from build123d import *

# Parameters (mm, degrees)
SKETCH1_W           = 40
SKETCH1_H           = 40
BOSS_EXTRUDE1_DEPTH = 3.18
SKETCH2_W           = 3.18
SKETCH2_H           = 10
BOSS_EXTRUDE2_DEPTH = 60
SKETCH3_W           = 3.18
SKETCH3_H           = 16
BOSS_EXTRUDE3_DEPTH = 36
FILLET1_R           = 10
FILLET2_R           = 8
FILLET3_R           = 5
FILLET4_R           = 4
SKETCH7_R           = 1
CUT_EXTRUDE2_DEPTH  = 3.18
SKETCH8_R           = 1
CUT_EXTRUDE3_DEPTH  = 3.18


with BuildPart() as part:
    # Sketch1 → Boss-Extrude1 (new body)
    with BuildSketch(Plane.XY):
        with Locations((50, 0)):
            Rectangle(SKETCH1_W, SKETCH1_H)
    extrude(amount=BOSS_EXTRUDE1_DEPTH)

    # Sketch2 → Boss-Extrude2 (add)
    with BuildSketch(Plane.ZY.offset(-30)):
        with Locations((1.59, 0)):
            Rectangle(SKETCH2_W, SKETCH2_H)
    extrude(amount=BOSS_EXTRUDE2_DEPTH)

    # Sketch3 → Boss-Extrude3 (add)
    with BuildSketch(Plane.ZY.offset(30)):
        with Locations((1.59, 0)):
            Rectangle(SKETCH3_W, SKETCH3_H)
    extrude(amount=BOSS_EXTRUDE3_DEPTH)

    # Fillet1
    fillet1_edges = [part.edges().sort_by_distance(p)[0] for p in [
        (70, -20, 1.59),
        (30, -20, 1.59),
        (30, 20, 1.59),
        (70, 20, 1.59),
    ]]
    fillet(fillet1_edges, radius=FILLET1_R)

    # Fillet2
    fillet2_edges = [part.edges().sort_by_distance(p)[0] for p in [
        (30, 5, 1.59),
        (30, -5, 1.59),
    ]]
    fillet(fillet2_edges, radius=FILLET2_R)

    # Fillet3
    # the kernel refuses this fillet: 5 mm, written as the material it takes off along each edge
    with BuildSketch(Plane(origin=(-30, 8, -11.456439237), x_dir=(-1, 0, 0), z_dir=(0, 0, 1))) as fillet3_piece_1:
        with BuildLine():
            CenterArc((4.582575695, 5), FILLET3_R, 203.578178478, 66.421821522)
            Line((0, 3), (-0.091651514, 2.96))
            ThreePointArc((-0.091651514, 2.96), (-0.1, 1.5), (-0.1, 0))
            Line((-0.1, 0), (0, -0.1))
            Line((0, -0.1), (4.582575695, -0.1))
            Line((4.582575695, -0.1), (4.582575695, 0))
        make_face()
    extrude(amount=26.092878475, mode=Mode.SUBTRACT)
    with BuildSketch(Plane(origin=(-66, 8, -12.5), x_dir=(0, -1, 0), z_dir=(0, 0, 1))) as fillet3_piece_2:
        with BuildLine():
            CenterArc((FILLET3_R, FILLET3_R), FILLET3_R, 180, 90)
            Line((0, FILLET3_R), (-FILLET3_R * 0.02, FILLET3_R))
            Line((-FILLET3_R * 0.02, FILLET3_R), (-FILLET3_R * 0.02, -FILLET3_R * 0.02))
            Line((-FILLET3_R * 0.02, -FILLET3_R * 0.02), (FILLET3_R, -FILLET3_R * 0.02))
            Line((FILLET3_R, -FILLET3_R * 0.02), (FILLET3_R, 0))
        make_face()
    extrude(amount=28.18, mode=Mode.SUBTRACT)
    with BuildSketch(Plane(origin=(-66, -8, 15.68), x_dir=(1, 0, 0), z_dir=(0, 0, -1))) as fillet3_piece_3:
        with BuildLine():
            CenterArc((FILLET3_R, -FILLET3_R), FILLET3_R, 90, 90)
            Line((0, -FILLET3_R), (-FILLET3_R * 0.02, -FILLET3_R))
            Line((-FILLET3_R * 0.02, -FILLET3_R), (-FILLET3_R * 0.02, FILLET3_R * 0.02))
            Line((-FILLET3_R * 0.02, FILLET3_R * 0.02), (FILLET3_R, FILLET3_R * 0.02))
            Line((FILLET3_R, FILLET3_R * 0.02), (FILLET3_R, 0))
        make_face()
    extrude(amount=28.18, mode=Mode.SUBTRACT)
    with BuildSketch(Plane(origin=(-30, -8, 14.636439237), x_dir=(0, 1, 0), z_dir=(0, 0, -1))) as fillet3_piece_4:
        with BuildLine():
            CenterArc((5, -4.582575695), FILLET3_R, 113.578178478, 66.421821522)
            Line((0, -4.582575695), (-0.1, -4.582575695))
            Line((-0.1, -4.582575695), (-0.1, 0))
            Line((-0.1, 0), (0, 0.1))
            ThreePointArc((0, 0.1), (1.5, 0.1), (2.96, 0.091651514))
            Line((2.96, 0.091651514), (3, 0))
        make_face()
    extrude(amount=26.092878475, mode=Mode.SUBTRACT)

    # Fillet4
    fillet4_edges = [part.edges().sort_by_distance(p)[0] for p in [
        (-30, -5, 1.59),
        (-30, 5, 1.59),
    ]]
    fillet(fillet4_edges, radius=FILLET4_R)

    # Sketch7 → Cut-Extrude2 (cut)
    with BuildSketch(Plane.XY.offset(3.18)):
        with Locations((63.45, 0)):
            Circle(SKETCH7_R)
        with Locations((36.55, 0)):
            Circle(SKETCH7_R)
        with Locations((50, 13.45)):
            Circle(SKETCH7_R)
        with Locations((50, -13.45)):
            Circle(SKETCH7_R)
    extrude(amount=-CUT_EXTRUDE2_DEPTH, mode=Mode.SUBTRACT)

    # Sketch8 → Cut-Extrude3 (cut)
    with BuildSketch(Plane.XY.offset(3.18)):
        with Locations((-32.97, -5)):
            Circle(SKETCH8_R)
        with Locations((-61, -5)):
            Circle(SKETCH8_R)
    extrude(amount=-CUT_EXTRUDE3_DEPTH, mode=Mode.SUBTRACT)


solid = part.part
Could you check a few things on this model? Use its own coordinates, in mm. A direction names the side the tool comes from. Give positions to 0.01 mm unless a question says otherwise; leave off trailing zeros. Order: outer loops, then holes, each group sorted by start corner. A loop starts at its lowest first (then second) coordinate and runs counter-clockwise, first axis right, second up.
1. Will these pins go through, and if not, where does the flat tip stop? P1, Ø1.6, axis at x = 63.45, y = 0, coming from the -Z side; P2, Ø1, axis at x = -39.5, z = 0.5, coming from the -Y side; P3, Ø1.6, axis at x = -2, z = 1.5, coming from the +Y side; P4, Ø1, axis at x = -3, z = 2.5, coming from the -Y side.
2. For faces 5 (the flat face through (-48, 8, 2)), 6 (the flat face through (-2, 5, 2)), 7 (the cylindrical face through (-32.51, -7.55, 1.61)), 8 (the flat face through (-48, -8, 2)), which set-ups out of +Z, -Z, +X, -X, +Y, -Y let a thin tool reach every point of the face, with its end or its side?
3. Suppose I cut it at C-C (x = -51.5). List the corners of the cut face in (y, z) for me.
4. Suppose I cut it at B-B (z = 2.15). Give the number of separate pieces and of enclosed holes in the cut face, plus the area to 3 significant figures.
5. We'd pull the mould along X, two halves only. Please class faces 1 (the cylindrical face through (-29.49, 5.34, 1.61)), 2 (the flat face through (50, -20, 2)), 3 (the cylindrical face through (-64, -7, 2)), 4 (the cylindrical face through (66.99, -17.15, 1.61)): pulls with the +X half, pulls with the -X half, needs draft (parallel to the pull), parting line crosses it, or undercut.
6. Suppose I cut it at A-A (y = -16). List the corners of the cut face in (x, z) for me, plus the area to 3 significant figures.
7. I need wall thicknesses on L1, parallel to Y at x = 50, z = 0.7; L2, parallel to Y at x = -61, z = 1.5; L3, parallel to Y at x = 5, z = 2.2. Which ranges of each line are inside material? Lowest first, please.
Solved:
1. P1: passes through
1. P2: stops at y = -8
1. P3: stops at y = 5
1. P4: stops at y = -5
2. face 5: +Z, -Z, -X, +Y
2. face 6: +Z, -Z, +Y
2. face 7: +Z, -Z, -Y
2. face 8: +Z, -Z, -X, -Y
3. outline: (-8, 0) - (8, 0) - (8, 3.18) - (-8, 3.18) - close
4. separate pieces: 1
4. enclosed holes: 6
4. area: 2,680 mm2
5. face 1: undercut
5. face 2: needs draft
5. face 3: pulls with the -X half
5. face 4: pulls with the +X half
6. outline: (32, 0) - (68, 0) - (68, 3.18) - (32, 3.18) - close
6. area: 114 mm2
7. L1: y = -20 to -14.45, -12.45 to 12.45, 14.45 to 20
7. L2: y = -8 to -6, -4 to 8
7. L3: y = -5 to 5
